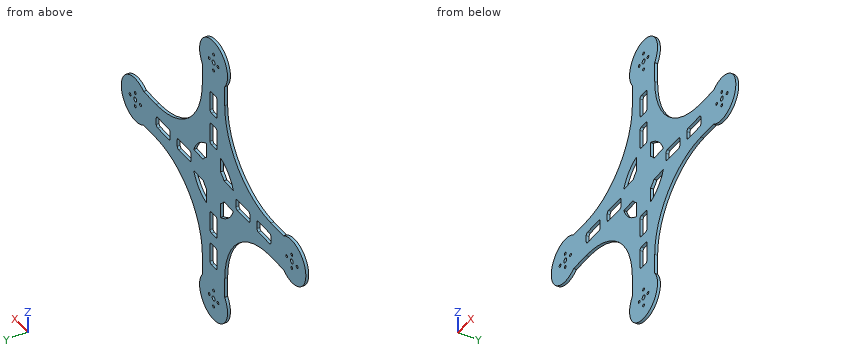
from build123d import *

# Parameters (mm, degrees)
SKETCH1_R           = 1.5875
SKETCH1_R_2         = 2.54
BOSS_EXTRUDE1_DEPTH = 3.175


with BuildPart() as part:
    # Sketch1 → Boss-Extrude1 (new body)
    with BuildSketch(Plane(origin=(0, 0, 0), x_dir=(1, 0, 0), z_dir=(0, 1, 0))):
        with BuildLine():
            ThreePointArc((106.34156313, 17.784127356), (65.70156313, -2.535872644), (106.34156313, -22.855872644))
            Line((106.34156313, -22.855872644), (129.095821507, -22.855872644))
            ThreePointArc((129.095821507, -22.855872644), (188.440282525, -47.437153249), (213.02156313, -106.781614267))
            Line((213.02156313, -106.781614267), (213.02156313, -129.535872644))
            ThreePointArc((213.02156313, -129.535872644), (233.34156313, -170.175872644), (253.66156313, -129.535872644))
            Line((253.66156313, -129.535872644), (253.66156313, -106.781614267))
            ThreePointArc((253.66156313, -106.781614267), (278.242843735, -47.437153249), (337.587304753, -22.855872644))
            Line((337.587304753, -22.855872644), (360.34156313, -22.855872644))
            ThreePointArc((360.34156313, -22.855872644), (400.98156313, -2.535872644), (360.34156313, 17.784127356))
            Line((360.34156313, 17.784127356), (337.587304753, 17.784127356))
            ThreePointArc((337.587304753, 17.784127356), (278.242843735, 42.365407962), (253.66156313, 101.70986898))
            Line((253.66156313, 101.70986898), (253.66156313, 124.464127356))
            ThreePointArc((253.66156313, 124.464127356), (233.34156313, 165.104127356), (213.02156313, 124.464127356))
            Line((213.02156313, 124.464127356), (213.02156313, 101.70986898))
            ThreePointArc((213.02156313, 101.70986898), (188.440282525, 42.365407962), (129.095821507, 17.784127356))
            Line((129.095821507, 17.784127356), (106.34156313, 17.784127356))
        make_face()
        with BuildLine():
            ThreePointArc((276.52156313, -8.885872644), (274.725511906, -8.141923868), (273.98156313, -6.345872644))
            Line((273.98156313, -6.345872644), (273.98156313, 1.274127356))
            ThreePointArc((273.98156313, 1.274127356), (274.725511906, 3.07017858), (276.52156313, 3.814127356))
            Line((276.52156313, 3.814127356), (296.84156313, 3.814127356))
            ThreePointArc((296.84156313, 3.814127356), (298.637614354, 3.07017858), (299.38156313, 1.274127356))
            Line((299.38156313, 1.274127356), (299.38156313, -6.345872644))
            ThreePointArc((299.38156313, -6.345872644), (298.637614354, -8.141923868), (296.84156313, -8.885872644))
            Line((296.84156313, -8.885872644), (276.52156313, -8.885872644))
        make_face(mode=Mode.SUBTRACT)
        with BuildLine():
            ThreePointArc((239.69156313, -66.035872644), (238.947614354, -67.831923868), (237.15156313, -68.575872644))
            Line((237.15156313, -68.575872644), (229.53156313, -68.575872644))
            ThreePointArc((229.53156313, -68.575872644), (227.735511906, -67.831923868), (226.99156313, -66.035872644))
            Line((226.99156313, -66.035872644), (226.99156313, -45.715872644))
            ThreePointArc((226.99156313, -45.715872644), (227.735511906, -43.91982142), (229.53156313, -43.175872644))
            Line((229.53156313, -43.175872644), (237.15156313, -43.175872644))
            ThreePointArc((237.15156313, -43.175872644), (238.947614354, -43.91982142), (239.69156313, -45.715872644))
            Line((239.69156313, -45.715872644), (239.69156313, -66.035872644))
        make_face(mode=Mode.SUBTRACT)
        with BuildLine():
            ThreePointArc((239.69156313, 40.644127356), (238.947614354, 38.848076132), (237.15156313, 38.104127356))
            Line((237.15156313, 38.104127356), (229.53156313, 38.104127356))
            ThreePointArc((229.53156313, 38.104127356), (227.735511906, 38.848076132), (226.99156313, 40.644127356))
            Line((226.99156313, 40.644127356), (226.99156313, 60.964127356))
            ThreePointArc((226.99156313, 60.964127356), (227.735511906, 62.76017858), (229.53156313, 63.504127356))
            Line((229.53156313, 63.504127356), (237.15156313, 63.504127356))
            ThreePointArc((237.15156313, 63.504127356), (238.947614354, 62.76017858), (239.69156313, 60.964127356))
            Line((239.69156313, 60.964127356), (239.69156313, 40.644127356))
        make_face(mode=Mode.SUBTRACT)
        with BuildLine():
            ThreePointArc((169.84156313, -8.885872644), (168.045511906, -8.141923868), (167.30156313, -6.345872644))
            Line((167.30156313, -6.345872644), (167.30156313, 1.274127356))
            ThreePointArc((167.30156313, 1.274127356), (168.045511906, 3.07017858), (169.84156313, 3.814127356))
            Line((169.84156313, 3.814127356), (190.16156313, 3.814127356))
            ThreePointArc((190.16156313, 3.814127356), (191.957614354, 3.07017858), (192.70156313, 1.274127356))
            Line((192.70156313, 1.274127356), (192.70156313, -6.345872644))
            ThreePointArc((192.70156313, -6.345872644), (191.957614354, -8.141923868), (190.16156313, -8.885872644))
            Line((190.16156313, -8.885872644), (169.84156313, -8.885872644))
        make_face(mode=Mode.SUBTRACT)
        with BuildLine():
            ThreePointArc((129.20156313, 1.274127356), (129.945511906, 3.07017858), (131.74156313, 3.814127356))
            Line((131.74156313, 3.814127356), (152.06156313, 3.814127356))
            ThreePointArc((152.06156313, 3.814127356), (153.857614354, 3.07017858), (154.60156313, 1.274127356))
            Line((154.60156313, 1.274127356), (154.60156313, -6.345872644))
            ThreePointArc((154.60156313, -6.345872644), (153.857614354, -8.141923868), (152.06156313, -8.885872644))
            Line((152.06156313, -8.885872644), (131.74156313, -8.885872644))
            ThreePointArc((131.74156313, -8.885872644), (129.945511906, -8.141923868), (129.20156313, -6.345872644))
            Line((129.20156313, -6.345872644), (129.20156313, 1.274127356))
        make_face(mode=Mode.SUBTRACT)
        with Locations(Location((91.10156313, 5.464127356, 0), (0, 0, 270))):
            Circle(SKETCH1_R, mode=Mode.SUBTRACT)
        with Locations(Location((100.60156313, -2.535872644, 0), (0, 0, 270))):
            Circle(SKETCH1_R, mode=Mode.SUBTRACT)
        with Locations(Location((91.10156313, -10.535872644, 0), (0, 0, 270))):
            Circle(SKETCH1_R, mode=Mode.SUBTRACT)
        with Locations(Location((91.10156313, -2.535872644, 0), (0, 0, 270))):
            Circle(SKETCH1_R_2, mode=Mode.SUBTRACT)
        with Locations(Location((81.60156313, -2.535872644, 0), (0, 0, 270))):
            Circle(SKETCH1_R, mode=Mode.SUBTRACT)
        with BuildLine():
            ThreePointArc((220.64156313, -38.456897128), (206.400794767, -29.476641007), (197.420538646, -15.235872644))
            Line((197.420538646, -15.235872644), (214.333943605, -15.235872644))
            ThreePointArc((214.333943605, -15.235872644), (217.177102112, -18.700333662), (220.64156313, -21.543492169))
            Line((220.64156313, -21.543492169), (220.64156313, -38.456897128))
        make_face(mode=Mode.SUBTRACT)
        with BuildLine():
            ThreePointArc((197.420538646, 10.164127356), (206.400794767, 24.404895719), (220.64156313, 33.385151841))
            Line((220.64156313, 33.385151841), (220.64156313, 16.471746881))
            ThreePointArc((220.64156313, 16.471746881), (217.177102112, 13.628588374), (214.333943605, 10.164127356))
            Line((214.333943605, 10.164127356), (197.420538646, 10.164127356))
        make_face(mode=Mode.SUBTRACT)
        with BuildLine():
            ThreePointArc((246.04156313, 33.385151841), (260.282331493, 24.404895719), (269.262587614, 10.164127356))
            Line((269.262587614, 10.164127356), (252.349182655, 10.164127356))
            ThreePointArc((252.349182655, 10.164127356), (249.506024148, 13.628588374), (246.04156313, 16.471746881))
            Line((246.04156313, 16.471746881), (246.04156313, 33.385151841))
        make_face(mode=Mode.SUBTRACT)
        with BuildLine():
            ThreePointArc((269.262587614, -15.235872644), (260.282331493, -29.476641007), (246.04156313, -38.456897128))
            Line((246.04156313, -38.456897128), (246.04156313, -21.543492169))
            ThreePointArc((246.04156313, -21.543492169), (249.506024148, -18.700333662), (252.349182655, -15.235872644))
            Line((252.349182655, -15.235872644), (269.262587614, -15.235872644))
        make_face(mode=Mode.SUBTRACT)
        with BuildLine():
            ThreePointArc((229.53156313, 76.204127356), (227.735511906, 76.948076132), (226.99156313, 78.744127356))
            Line((226.99156313, 78.744127356), (226.99156313, 99.064127356))
            ThreePointArc((226.99156313, 99.064127356), (227.735511906, 100.86017858), (229.53156313, 101.604127356))
            Line((229.53156313, 101.604127356), (237.15156313, 101.604127356))
            ThreePointArc((237.15156313, 101.604127356), (238.947614354, 100.86017858), (239.69156313, 99.064127356))
            Line((239.69156313, 99.064127356), (239.69156313, 78.744127356))
            ThreePointArc((239.69156313, 78.744127356), (238.947614354, 76.948076132), (237.15156313, 76.204127356))
            Line((237.15156313, 76.204127356), (229.53156313, 76.204127356))
        make_face(mode=Mode.SUBTRACT)
        with Locations(Location((233.34156313, 149.204127356, 0), (0, 0, 270))):
            Circle(SKETCH1_R, mode=Mode.SUBTRACT)
        with Locations(Location((225.34156313, 139.704127356, 0), (0, 0, 270))):
            Circle(SKETCH1_R, mode=Mode.SUBTRACT)
        with Locations(Location((233.34156313, 130.204127356, 0), (0, 0, 270))):
            Circle(SKETCH1_R, mode=Mode.SUBTRACT)
        with Locations(Location((233.34156313, 139.704127356, 0), (0, 0, 270))):
            Circle(SKETCH1_R_2, mode=Mode.SUBTRACT)
        with Locations(Location((241.34156313, 139.704127356, 0), (0, 0, 270))):
            Circle(SKETCH1_R, mode=Mode.SUBTRACT)
        with BuildLine():
            ThreePointArc((237.15156313, -81.275872644), (238.947614354, -82.01982142), (239.69156313, -83.815872644))
            Line((239.69156313, -83.815872644), (239.69156313, -104.135872644))
            ThreePointArc((239.69156313, -104.135872644), (238.947614354, -105.931923868), (237.15156313, -106.675872644))
            Line((237.15156313, -106.675872644), (229.53156313, -106.675872644))
            ThreePointArc((229.53156313, -106.675872644), (227.735511906, -105.931923868), (226.99156313, -104.135872644))
            Line((226.99156313, -104.135872644), (226.99156313, -83.815872644))
            ThreePointArc((226.99156313, -83.815872644), (227.735511906, -82.01982142), (229.53156313, -81.275872644))
            Line((229.53156313, -81.275872644), (237.15156313, -81.275872644))
        make_face(mode=Mode.SUBTRACT)
        with Locations(Location((233.34156313, -135.275872644, 0), (0, 0, 270))):
            Circle(SKETCH1_R, mode=Mode.SUBTRACT)
        with Locations(Location((225.34156313, -144.775872644, 0), (0, 0, 270))):
            Circle(SKETCH1_R, mode=Mode.SUBTRACT)
        with Locations(Location((233.34156313, -154.275872644, 0), (0, 0, 270))):
            Circle(SKETCH1_R, mode=Mode.SUBTRACT)
        with Locations(Location((233.34156313, -144.775872644, 0), (0, 0, 270))):
            Circle(SKETCH1_R_2, mode=Mode.SUBTRACT)
        with Locations(Location((241.34156313, -144.775872644, 0), (0, 0, 270))):
            Circle(SKETCH1_R, mode=Mode.SUBTRACT)
        with BuildLine():
            Line((334.94156313, -8.885872644), (314.62156313, -8.885872644))
            ThreePointArc((314.62156313, -8.885872644), (312.825511906, -8.141923868), (312.08156313, -6.345872644))
            Line((312.08156313, -6.345872644), (312.08156313, 1.274127356))
            ThreePointArc((312.08156313, 1.274127356), (312.825511906, 3.07017858), (314.62156313, 3.814127356))
            Line((314.62156313, 3.814127356), (334.94156313, 3.814127356))
            ThreePointArc((334.94156313, 3.814127356), (336.737614354, 3.07017858), (337.48156313, 1.274127356))
            Line((337.48156313, 1.274127356), (337.48156313, -6.345872644))
            ThreePointArc((337.48156313, -6.345872644), (336.737614354, -8.141923868), (334.94156313, -8.885872644))
        make_face(mode=Mode.SUBTRACT)
        with Locations(Location((385.08156313, -2.535872644, 0), (0, 0, 270))):
            Circle(SKETCH1_R, mode=Mode.SUBTRACT)
        with Locations(Location((375.58156313, -10.535872644, 0), (0, 0, 270))):
            Circle(SKETCH1_R, mode=Mode.SUBTRACT)
        with Locations(Location((375.58156313, -2.535872644, 0), (0, 0, 270))):
            Circle(SKETCH1_R_2, mode=Mode.SUBTRACT)
        with Locations(Location((366.08156313, -2.535872644, 0), (0, 0, 270))):
            Circle(SKETCH1_R, mode=Mode.SUBTRACT)
        with Locations(Location((375.58156313, 5.464127356, 0), (0, 0, 270))):
            Circle(SKETCH1_R, mode=Mode.SUBTRACT)
    extrude(amount=BOSS_EXTRUDE1_DEPTH)


solid = part.part
Work out the finished part from the listing and answer in its coordinate system (mm). Give positions to 0.01 mm unless a question says otherwise; leave off trailing zeros. Loops run counter-clockwise (first coordinate to the right, second up) from the corner with the lowest first, then second, coordinate; pieces in that order, holes last. Notation, with made-up numbers: (49.25, 13) - (96.25, 13) arc R21 cw to (96.25, 41) - close; hole circle Ø9 at (-17.75, 34). An arc over 180 degrees is marked (long way). Answer in a Markdown table with one row per item.
(1) Section C-C (z = 121) is taken. Give the vertices of the cut face in (x, y) (3 decimals), and give its area (3 significant figures).
Results list:
| item | result |
|---|---|
| outline | (213.022, 0) - (253.662, 0) - (253.662, 3.175) - (213.022, 3.175) - close |
| area | 129 mm² |
(2) Consider L1, parallel to Z at x = 249.5, y = 0.6; L2, parallel to X at y = 0.6, z = -26.5; L3, parallel to X at y = 1.95, z = -120. Determine where each line is inside the solid, lowest interval first. Write a range as [from, to].
Results list:
| item | result |
|---|---|
| L1 | z = [-159.3, -31.97], [-13.63, 18.71], [37.04, 164.37] |
| L2 | x = [166.34, 208.67], [220.64, 246.04], [258.01, 300.34] |
| L3 | x = [213.02, 253.66] |
(3) Flat-ended cylindrical pins translate along their axes: pin 1 Ø1.5 at (x, y) = (352.5, 3) entering from +Z; pin 2 Ø1 at (x, y) = (203.5, 1.5) entering from +Z; pin 3 Ø1.6 at (y, z) = (2, 122.5) entering from +X. Find the tip coordinate at first contact, or state that the pin passes through.
Results list:
| item | result |
|---|---|
| pin 1 | stops at z = 22.86 |
| pin 2 | stops at z = 68.93 |
| pin 3 | stops at x = 253.66 |
(4) Section B-B (x = 202.5) is taken. Give the vertices of the cut face in (y, z) (3 decimals), and give its area (3 significant figures).
Results list:
| item | result |
|---|---|
| outline | (0, -61.024) - (3.175, -61.024) - (3.175, -19.834) - (0, -19.834) - close; (0, -10.164) - (3.175, -10.164) - (3.175, 15.236) - (0, 15.236) - close; (0, 24.906) - (3.175, 24.906) - (3.175, 66.096) - (0, 66.096) - close |
| area | 342 mm² |
(5) Section A-A (x = 287.5) is taken. Give the vertices of the cut face in (y, z) (3 decimals), and give its area (3 significant figures).
Results list:
| item | result |
|---|---|
| outline | (0, -34.369) - (3.175, -34.369) - (3.175, -3.814) - (0, -3.814) - close; (0, 8.886) - (3.175, 8.886) - (3.175, 39.441) - (0, 39.441) - close |
| area | 194 mm² |
(6) Section D-D (y = 1.25) is taken. State how many separate pieces and enclosed holes the cut face has, and give its area (3 significant figures).
Results list:
| item | result |
|---|---|
| separate pieces | 1 |
| enclosed holes | 32 |
| area | 27,900 mm² |
